The listing builds one solid part. Answer for the finished solid, in the listing's coordinates (mm). Coordinates: 2 decimals unless noted, no trailing zeros. Loops run counter-clockwise (first coordinate to the right, second up) from the corner with the lowest first, then second, coordinate; pieces in that order, holes last. Notation, with made-up numbers: M 63,-2 L 102,-2 A19 cw 102,7 Z; hole C -26,-18.5 d11. An arc over 180 degrees is marked long. Answer as a JSON object with one key per item and string values. Group by question number.
1. A cutting plane is placed at B-B on x = 5. Give the vertices of the cut face in (y, z), and give its area (3 significant figures).
2. Straight lines are drawn through the part: L1, parallel to X at y = 7.25, z = 18.5; L2, parallel to Y at x = 7, z = 24. For each, find the intervals that lie inside material, in ascending order.
3. A cutting plane is placed at A-A on y = 8. Give the vertices of the cut face in (x, z).
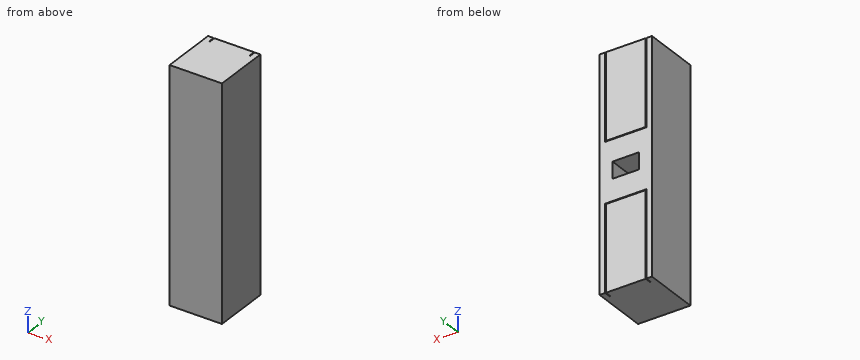
from build123d import *

# Parameters (mm, degrees)
SKETCH1_W           = 7.9
SKETCH1_H           = 8.5
BOSS_EXTRUDE1_DEPTH = 35
CUT_EXTRUDE1_DEPTH  = 1
SKETCH3_W           = 4
SKETCH3_H           = 2.5
CUT_EXTRUDE2_DEPTH  = 3.5


with BuildPart() as part:
    # Sketch1 → Boss-Extrude1 (new body)
    with BuildSketch(Plane.XY):
        with Locations((3.95, 4.25)):
            Rectangle(SKETCH1_W, SKETCH1_H)
    extrude(amount=BOSS_EXTRUDE1_DEPTH)

    # Sketch2 → Cut-Extrude1 (cut)
    with BuildSketch(Plane(origin=(0, 8.5, 0), x_dir=(1, 0, 0), z_dir=(0, 1, 0))):
        Polygon((0.85, -35), (0.95, -35), (0.95, -22.1), (6.95, -22.1), (6.95, -35), (7.05, -35), (7.05, -22), (0.85, -22), align=None)
        Polygon((6.95, 0), (7.05, 0), (7.05, -13), (0.85, -13), (0.85, 0), (0.95, 0), (0.95, -12.9), (6.95, -12.9), align=None)
    extrude(amount=-CUT_EXTRUDE1_DEPTH, mode=Mode.SUBTRACT)

    # Sketch3 → Cut-Extrude2 (cut)
    with BuildSketch(Plane(origin=(0, 8.5, 0), x_dir=(1, 0, 0), z_dir=(0, 1, 0))):
        with Locations((3.95, -17.5)):
            Rectangle(SKETCH3_W, SKETCH3_H)
    extrude(amount=-CUT_EXTRUDE2_DEPTH, mode=Mode.SUBTRACT)


solid = part.part
From the geometry:
{
 "1": {"outline": "M 0,0 L 8.5,0 L 8.5,12.9 L 7.5,12.9 L 7.5,13 L 8.5,13 L 8.5,16.25 L 5,16.25 L 5,18.75 L 8.5,18.75 L 8.5,22 L 7.5,22 L 7.5,22.1 L 8.5,22.1 L 8.5,35 L 0,35 Z", "area": "289 mm²"},
 "2": {"L1": "x = 0 to 1.95, 5.95 to 7.9", "L2": "y = 0 to 7.5"},
 "3": {"outline": "M 0,0 L 0.85,0 L 0.85,13 L 7.05,13 L 7.05,0 L 7.9,0 L 7.9,35 L 7.05,35 L 7.05,22 L 0.85,22 L 0.85,35 L 0,35 Z; M 0.95,0 L 6.95,0 L 6.95,12.9 L 0.95,12.9 Z; M 0.95,22.1 L 6.95,22.1 L 6.95,35 L 0.95,35 Z; hole M 1.95,16.25 L 5.95,16.25 L 5.95,18.75 L 1.95,18.75 Z"}
}
